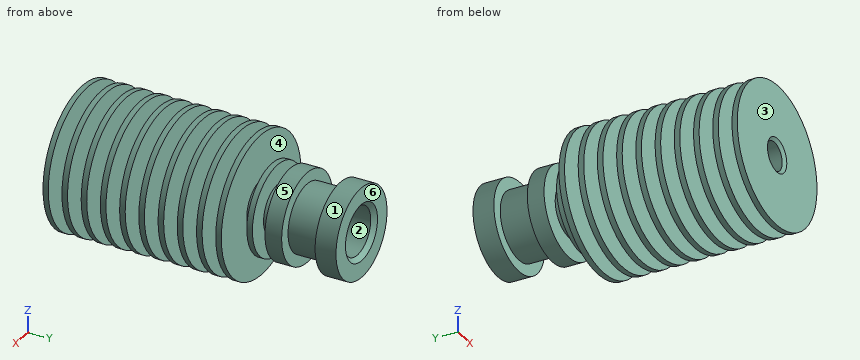
from build123d import *

# Parameters (mm, degrees)
SZKIC2_W                          = 2
SZKIC2_H                          = 6
SZKIC3_W                          = 3.5
SZKIC3_H                          = 2.25
SZKIC3_H_2                        = 2
SZKIC4_W                          = 8
SZKIC4_H                          = 2.45
SZKIC5_W                          = 6.5
SZKIC5_H                          = 2.45
SZKIC6_W                          = 5.5
SZKIC6_H                          = 2.45
OTW_R_GWINTOWANY_M61_D            = 5
OTW_R_GWINTOWANY_M61_DEPTH        = 27.5
OTW_R_GWINTOWANY_M61_CSINK_D      = 6.05
OTW_R_GWINTOWANY_M61_CSINK_ANGLE  = 90
OTW_R_GWINTOWANY_M61_TIP          = 1.502151548
OTW_R_GWINTOWANY_M102_D           = 8.5
OTW_R_GWINTOWANY_M102_DEPTH       = 10
OTW_R_GWINTOWANY_M102_CSINK_D     = 10.05
OTW_R_GWINTOWANY_M102_CSINK_ANGLE = 90
OTW_R_GWINTOWANY_M102_TIP         = 2.553657631
WYTNIJ_WYCI_GNI_CIE1_REACH        = 55.033
SZKIC14_R                         = 0.95


with BuildPart() as part:
    # Szkic1 → Obrót1 (revolve)
    with BuildSketch(Plane.XY, mode=Mode.PRIVATE) as obr_t1_sk:
        Polygon((0, 0), (-12.5, 0), (-12.5, 32), (-8, 32), (-8, 50), (0, 50), align=None)
    revolve(obr_t1_sk.sketch.rotate(Axis((0, 50, 0), (0, -1, 0)), 270), axis=Axis((0, 50, 0), (0, -1, 0)))

    # Szkic2 → Wycięcie-obrót1 (revolve, cut)
    with BuildSketch(Plane.XY, mode=Mode.PRIVATE) as wyci_cie_obr_t1_sk:
        with Locations((-7, 43.25)):
            Rectangle(SZKIC2_W, SZKIC2_H)
    revolve(wyci_cie_obr_t1_sk.sketch.rotate(Axis((0, 46.25, 0), (0, -1, 0)), 270), axis=Axis((0, 46.25, 0), (0, -1, 0)), mode=Mode.SUBTRACT)

    # Szkic3 → Wycięcie-obrót2 (revolve, cut)
    with BuildSketch(Plane.XY, mode=Mode.PRIVATE) as wyci_cie_obr_t2_sk:
        with Locations((-6.25, 36.125)):
            Rectangle(SZKIC3_W, SZKIC3_H)
        with Locations((-6.25, 33)):
            Rectangle(SZKIC3_W, SZKIC3_H_2)
    revolve(wyci_cie_obr_t2_sk.sketch.rotate(Axis((0, 32, 0), (0, 1, 0)), 270), axis=Axis((0, 32, 0), (0, 1, 0)), mode=Mode.SUBTRACT)

    # Szkic4 → Wycięcie-obrót3 (revolve, cut)
    with BuildSketch(Plane.XY, mode=Mode.PRIVATE) as wyci_cie_obr_t3_sk:
        with Locations((-8.5, 29.775)):
            Rectangle(SZKIC4_W, SZKIC4_H)
        with Locations((-8.5, 26.325)):
            Rectangle(SZKIC4_W, SZKIC4_H)
        with Locations((-8.5, 22.875)):
            Rectangle(SZKIC4_W, SZKIC4_H)
    revolve(wyci_cie_obr_t3_sk.sketch.rotate(Axis((0, 0, 0), (0, 1, 0)), 270), axis=Axis((0, 0, 0), (0, 1, 0)), mode=Mode.SUBTRACT)

    # Szkic5 → Wycięcie-obrót4 (revolve, cut)
    with BuildSketch(Plane.XY, mode=Mode.PRIVATE) as wyci_cie_obr_t4_sk:
        with Locations((-9.25, 19.425)):
            Rectangle(SZKIC5_W, SZKIC5_H)
    revolve(wyci_cie_obr_t4_sk.sketch.rotate(Axis((0, 50, 0), (0, 1, 0)), 270), axis=Axis((0, 50, 0), (0, 1, 0)), mode=Mode.SUBTRACT)

    # Szkic6 → Wycięcie-obrót5 (revolve, cut)
    with BuildSketch(Plane.XY, mode=Mode.PRIVATE) as wyci_cie_obr_t5_sk:
        with Locations((-9.75, 15.975)):
            Rectangle(SZKIC6_W, SZKIC6_H)
        with Locations((-9.75, 12.525)):
            Rectangle(SZKIC6_W, SZKIC6_H)
        with Locations((-9.75, 9.075)):
            Rectangle(SZKIC6_W, SZKIC6_H)
        with Locations((-9.75, 5.625)):
            Rectangle(SZKIC6_W, SZKIC6_H)
        with Locations((-9.75, 2.175)):
            Rectangle(SZKIC6_W, SZKIC6_H)
    revolve(wyci_cie_obr_t5_sk.sketch.rotate(Axis((0, 50, 0), (0, 1, 0)), 270), axis=Axis((0, 50, 0), (0, 1, 0)), mode=Mode.SUBTRACT)

    # Otwór gwintowany M61
    with Locations(Plane(origin=(0, 0, 0), x_dir=(-1, 0, 0), z_dir=(0, -1, 0))):
        with Locations((0, 0)):
            CounterSinkHole(OTW_R_GWINTOWANY_M61_D / 2, OTW_R_GWINTOWANY_M61_CSINK_D / 2, depth=OTW_R_GWINTOWANY_M61_DEPTH, counter_sink_angle=OTW_R_GWINTOWANY_M61_CSINK_ANGLE)
            with Locations((0, 0, -(OTW_R_GWINTOWANY_M61_DEPTH + OTW_R_GWINTOWANY_M61_TIP / 2))):  # 118° drill point
                Cone(0, OTW_R_GWINTOWANY_M61_D / 2, OTW_R_GWINTOWANY_M61_TIP, mode=Mode.SUBTRACT)

    # Otwór gwintowany M102
    with Locations(Plane(origin=(0, 50, 0), x_dir=(1, 0, 0), z_dir=(0, 1, 0))):
        with Locations((0, 0)):
            CounterSinkHole(OTW_R_GWINTOWANY_M102_D / 2, OTW_R_GWINTOWANY_M102_CSINK_D / 2, depth=OTW_R_GWINTOWANY_M102_DEPTH, counter_sink_angle=OTW_R_GWINTOWANY_M102_CSINK_ANGLE)
            with Locations((0, 0, -(OTW_R_GWINTOWANY_M102_DEPTH + OTW_R_GWINTOWANY_M102_TIP / 2))):  # 118° drill point
                Cone(0, OTW_R_GWINTOWANY_M102_D / 2, OTW_R_GWINTOWANY_M102_TIP, mode=Mode.SUBTRACT)

    # Wytnij-wyciągnięcie1: up to this cone (the profile starts outside it)
    wytnij_wyci_gni_cie1_end = Plane(origin=(0, 50, 0), z_dir=(0, -1, 0)).offset(20.997849452) * Cone(1.664e-06, 57.47614414, 34.535150548, align=(Align.CENTER, Align.CENTER, Align.MIN), mode=Mode.PRIVATE)
    # Szkic14 → Wytnij-wyciągnięcie1 (cut, up to the surface)
    with BuildSketch(Plane(origin=(0, 50, 0), x_dir=(1, 0, 0), z_dir=(0, 1, 0)), mode=Mode.PRIVATE) as wytnij_wyci_gni_cie1_sk1:
        with Locations(Location((0, 0, 0), (0, 0, 270))):
            Circle(SZKIC14_R)
    wytnij_wyci_gni_cie1_tool1 = extrude(wytnij_wyci_gni_cie1_sk1.sketch, amount=-WYTNIJ_WYCI_GNI_CIE1_REACH, mode=Mode.PRIVATE) - wytnij_wyci_gni_cie1_end
    add(wytnij_wyci_gni_cie1_tool1.solids().sort_by_distance((0, 50, 0))[0], mode=Mode.SUBTRACT)


solid = part.part
Could you check a few things on this model? Use its own coordinates, in mm. Face numbers are marked on the shaded views. A direction names the side the tool comes from. Round coordinates to 2 decimals unless told otherwise and drop trailing zeros. Write each loop counter-clockwise with the first axis right and the second up, starting at its lowest first coordinate (ties: lowest second). Pieces come first, ordered by that corner, then holes. Notation, with made-up numbers: (66, 11.25) -> (99, 11.25) arc R14 ccw to (99, 29.25) -> close; hole circle Ø1 at (3.25, -11). An arc over 180 degrees is marked (long way). Use a Markdown table: item, result.
1. If we section it at B-B (z = 8.5): State how many separate pieces and enclosed holes the cut face has, then the cut area to 3 significant figures.
Answer key:
| item | result |
|---|---|
| separate pieces | 10 |
| enclosed holes | 0 |
| area | 182 mm^2 |
2. Which directions (+Z, -Z, +X, -X, +Y, -Y) give clear straight access to the entire face, cutting with the end or side of a thin tool? Please do the marked faces 4, 5 and 6.
Answer key:
| item | result |
|---|---|
| face 4 | none |
| face 5 | +Y |
| face 6 | +Z, -Z, +X, -X, +Y |
3. We'd pull the mould along Z, two halves only. Please class the marked faces 1, 2 and 3: +Z half, -Z half, draft (parallel to the pull), parting line (faces both ways), or undercut.
Answer key:
| item | result |
|---|---|
| face 1 | parting line |
| face 2 | undercut |
| face 3 | draft |
4. Please list where these lines run through material, in increasing order: probe 1 along Y at (x, z) = (1.25, 5); probe 2 along X at (y, z) = (28.5, -0.75); probe 3 along Y at (x, z) = (-2, 4.25).
Answer key:
| item | result |
|---|---|
| probe 1 | y = 0 to 21.65, 24.1 to 25.1, 27.55 to 28.55, 31 to 32, 34 to 35, 37.25 to 50 |
| probe 2 | x = -12.48 to -0.58, 0.58 to 12.48 |
| probe 3 | y = 0 to 21.65, 24.1 to 25.1, 27.55 to 28.55, 31 to 32, 34 to 35, 37.25 to 49.67 |
5. For pin 1 Ø1.5 at (x, y) = (-0.5, 16) entering from +Z; pin 2 Ø1.5 at (y, z) = (20.5, -9) entering from -X, each with a flat end and sliding along its axis, tell me the tip position at first contact or that it passes through.
Answer key:
| item | result |
|---|---|
| pin 1 | stops at z = 7 |
| pin 2 | stops at x = -9.38 |
6. If we section it at A-A (y = 27): List the corners of the cut face in (x, z) for me, then the cut area to 3 significant figures.
Answer key:
| item | result |
|---|---|
| outline | circle Ø9 at (0, 0); hole circle Ø5 at (0, 0) |
| area | 44.0 mm^2 |
